The model under review builds one solid part; all positions refer to its coordinate system, in mm. Round coordinates to 2 decimals unless told otherwise and drop trailing zeros. Order: outer loops, then holes, each group sorted by start corner. A loop starts at its lowest first (then second) coordinate and runs counter-clockwise, first axis right, second up. Notation, with made-up numbers: M 38.25,7.5 L 97.25,7.5 A13 cw 97.25,28.5 Z; hole C 38,84 d11. An arc over 180 degrees is marked long. Answer as CSV lines item,"result". Start each with the question number.
from build123d import *

# Parameters (mm, degrees)
F1_DEPTH = 70.866
F2_R     = 34.339774


with BuildPart() as f1:
    # F0 (on Top) → F1 (new body)
    with BuildSketch(Plane.XY):
        Polygon((45.39609, 30.624349), (-46.83724, 30.624349), (-46.83724, 28.46263), (-46.83724, -36.38893), (45.39609, -36.38893), align=None)
    extrude(amount=F1_DEPTH)

    # F2
    f2_edges = [f1.edges().sort_by_distance(p)[0] for p in [
        (45.39609, 30.624349, 35.433),
        (-46.83724, 30.624349, 35.433),
        (-0.720575, 30.624349, 0),
        (-0.720575, 30.624349, 70.866),
    ]]
    fillet(f2_edges, radius=F2_R)


solid = f1.part
Item 1: Consider section C-C (y = 4). State the section outline as (x, z) points, and give its area (3 significant figures).
Item 2: Consider section A-A (x = 7). State the section outline as (y, z) points.
Item 3: Wall thickness on probe 1 along Y at (x, z) = (-24, 30); probe 2 along Y at (x, z) = (-6, 15.5); probe 3 along X at (y, z) = (9.5, 57): over which ranges is each line inside the solid? List them lowest first. Write a range as [from, to].
Item 4: Consider section B-B (z = 43). State the section outline as (x, y) points, and give its area (3 significant figures).
Item 5: For pin 1 (1 mm diameter, centred on y = 1.5, z = 50.5, fed in from -X); pin 2 (3 mm diameter, centred on x = -2, y = 23, fed in from +Z); pin 3 (12 mm diameter, centred on x = 19, y = -16.5, fed in from -Z); pin 4 (6 mm diameter, centred on y = 9.5, z = 20.5, fed in from -X), all flat-tipped, find the tip position at first contact; note any pin that passes through.
Reported:
1,outline,"M -45.96,0.88 L 44.52,0.88 L 44.52,69.99 L -45.96,69.99 Z"
1,area,"6,250 mm²"
2,outline,"M -36.39,0 L -3.72,0 A34.34 ccw 30.62,34.34 L 30.62,36.53 A34.34 ccw -3.72,70.87 L -36.39,70.87 Z"
3,probe 1,"y = [-36.39, 28.64]"
3,probe 2,"y = [-36.39, 24.99]"
3,probe 3,"x = [-44.19, 42.75]"
4,outline,"M -46.84,-36.39 L 45.4,-36.39 L 45.4,-3.72 A34.34 ccw 17.53,30.01 L -18.97,30.01 A34.34 ccw -46.84,-3.72 Z"
4,area,"5,650 mm²"
5,pin 1,"stops at x = -46.51"
5,pin 2,"stops at z = 59.84"
5,pin 3,"stops at z = 0"
5,pin 4,"stops at x = -45.28"
